The listing builds one solid part. Answer for the finished solid, in the listing's coordinates (mm). Coordinates: 2 decimals unless noted, no trailing zeros. Order: outer loops, then holes, each group sorted by start corner. A loop starts at its lowest first (then second) coordinate and runs counter-clockwise, first axis right, second up. Notation, with made-up numbers: (17, 49.25) - (27, 49.25) arc R11 ccw to (27, 62.25) - close; hole circle Ø4 at (67, -23.75). An arc over 180 degrees is marked (long way). Use a Markdown table: item, result. Add a question column.
Item 1: A flat-ended cylindrical pin translates along its axis: P1, Ø3.5, axis at x = 6, y = -6, coming from the -Z side. Find the tip coordinate at first contact, or state that the pin passes through.
Item 2: Find the intervals of material crossed by line 1 along Y through (x, z) = (6, 0.9); line 2 along Y through (x, z) = (7, 1.7); line 3 along Y through (x, z) = (56.5, 1.4), in increasing order.
Item 3: The part is cut by section B-B, the plane z = 2.25. Give the vertices of the cut face in (x, y).
Item 4: The part is cut by section A-A, the plane y = -32. Give the vertices of the cut face in (x, z), then the cut area to 3 significant figures.
Item 5: The mould has two halves that part along X. Classify faces 1 (the cylindrical face through (55.064, -31.932, 0.74)), 2 (the cylindrical face through (4.45, -5.93, 0.74)), 3 (the flat face through (34, -32, 0)), 4 (the cylindrical face through (1.804, -1.711, 0.493)): released by +X, released by -X, zero draft, split by the parting line, or undercut.
from build123d import *

# Parameters (mm, degrees)
SKETCH_R     = 1.55
PAD_DEPTH    = 3
CHAMFER_SIZE = 1.5
FILLET_R     = 2


with BuildPart() as part:
    # Sketch → Pad (new body)
    with BuildSketch(Plane.XY):
        with BuildLine():
            ThreePointArc((6, 0), (1.757359, -1.757359), (0, -6))
            Line((0, -58), (0, -6))
            ThreePointArc((0, -58), (1.757359, -62.242641), (6, -64))
            Line((63, -64), (6, -64))
            ThreePointArc((63, -64), (67.242641, -62.242641), (69, -58))
            Line((69, -6), (69, -58))
            ThreePointArc((69, -6), (67.242641, -1.757359), (63, 0))
            Line((6, 0), (63, 0))
        make_face()
        with Locations((6, -6)):
            Circle(SKETCH_R, mode=Mode.SUBTRACT)
        with Locations((6, -58)):
            Circle(SKETCH_R, mode=Mode.SUBTRACT)
        with Locations((56.61235, -32)):
            Circle(SKETCH_R, mode=Mode.SUBTRACT)
    extrude(amount=PAD_DEPTH)

    # Chamfer
    chamfer_edges = [part.edges().sort_by_distance(p)[0] for p in [
        (4.45, -6, 3),
        (4.45, -58, 3),
        (55.06235, -32, 3),
    ]]
    chamfer(chamfer_edges, length=CHAMFER_SIZE)

    # Fillet
    fillet_edges = [part.edges().sort_by_distance(p)[0] for p in [
        (69, -32, 3),
    ]]
    fillet(fillet_edges, radius=FILLET_R)


solid = part.part
Solution:
| question | item | result |
|---|---|---|
| 1 | P1 | stops at z = 0 |
| 2 | line 1 | y = -64 to -59.55, -56.45 to -7.55, -4.45 to 0 |
| 2 | line 2 | y = -63.87 to -59.44, -56.56 to -7.44, -4.56 to -0.13 |
| 2 | line 3 | y = -63.96 to -33.55, -30.45 to -0.04 |
| 3 | outline | (0.44, -58) arc R5.56 ccw to (6, -63.56) - (63, -63.56) arc R5.56 ccw to (68.56, -58) - (68.56, -6) arc R5.56 ccw to (63, -0.44) - (6, -0.44) arc R5.56 ccw to (0.44, -6) - close; hole circle Ø4.6 at (6, -58); hole circle Ø4.6 at (6, -6); hole circle Ø4.6 at (56.61, -32) |
| 4 | outline | (0, 0) - (55.06, 0) - (55.06, 1.5) - (53.56, 3) - (2, 3) arc R2 ccw to (0, 1) - close; (58.16, 0) - (69, 0) - (69, 1) arc R2 ccw to (67, 3) - (59.66, 3) - (58.16, 1.5) - close |
| 4 | area | 194 mm2 |
| 5 | face 1 | undercut |
| 5 | face 2 | undercut |
| 5 | face 3 | zero draft |
| 5 | face 4 | released by -X |
